```python
from build123d import *

# Parameters (mm, degrees)
BASE_SKETCH_W            = 254
BASE_SKETCH_H            = 304.8
BASE_DEPTH               = 25.4
RIGHT_TRIANGLE_DEPTH     = 25.4
LEFT_TRIANGLE_DEPTH      = 25.4
SUPPORT_BEAMS_SKETCH_W   = 114.3
SUPPORT_BEAMS_SKETCH_H   = 203.2
SUPPORT_BEAMS_SKETCH_W_2 = 50.8
SUPPORT_BEAMS_SKETCH_W_3 = 88.9
SUPPORT_BEAMS_DEPTH      = 25.4
FILLET1_R                = 12.7
TOP_PLATE_SKETCH_W       = 228.6
TOP_PLATE_SKETCH_H       = 254
TOP_PLATE_DEPTH          = 25.4
FILLET4_R                = 2.54
CUT_EXTRUDE1_DEPTH       = 229.6
FILLET6_R                = 6.35


with BuildPart() as part:
    # Base Sketch → Base (new body)
    with BuildSketch(Plane(origin=(0, 0, 0), x_dir=(0, 0, -1), z_dir=(1, 0, 0))):
        Rectangle(BASE_SKETCH_W, BASE_SKETCH_H)
    extrude(amount=BASE_DEPTH)

    # Right Triangle Sketch → Right Triangle (add)
    with BuildSketch(Plane.XY.offset(101.6)):
        Polygon((0, 152.4), (876.3, 152.4), (876.3, 127), (50.8, -152.4), (0, -152.4), align=None)
    extrude(amount=-RIGHT_TRIANGLE_DEPTH)

    # Left Triangle Sketch → Left Triangle (add)
    with BuildSketch(Plane(origin=(0, 0, -101.6), x_dir=(-1, 0, 0), z_dir=(0, 0, -1))):
        Polygon((0, 152.4), (-876.3, 152.4), (-876.3, 127), (-50.8, -152.4), (0, -152.4), align=None)
    extrude(amount=-LEFT_TRIANGLE_DEPTH)

    # Support Beams Sketch → Support Beams (add)
    with BuildSketch(Plane(origin=(0, 152.4, 0), x_dir=(1, 0, 0), z_dir=(0, 1, 0))):
        with Locations((57.15, 0)):
            Rectangle(SUPPORT_BEAMS_SKETCH_W, SUPPORT_BEAMS_SKETCH_H)
        with Locations((304.8, 0)):
            Rectangle(SUPPORT_BEAMS_SKETCH_W_2, SUPPORT_BEAMS_SKETCH_H)
        with Locations((831.85, 0)):
            Rectangle(SUPPORT_BEAMS_SKETCH_W_3, SUPPORT_BEAMS_SKETCH_H)
    extrude(amount=-SUPPORT_BEAMS_DEPTH)

    # Fillet1
    fillet1_edges = [part.edges().sort_by_distance(p)[0] for p in [
        (279.4, 139.7, 76.2),
        (330.2, 139.7, 76.2),
        (304.8, 127, 76.2),
        (304.8, 127, -76.2),
        (279.4, 139.7, -76.2),
        (330.2, 139.7, -76.2),
        (787.4, 139.7, 76.2),
        (831.85, 127, 76.2),
        (831.85, 127, -76.2),
        (787.4, 139.7, -76.2),
        (25.4, 0, 101.6),
        (876.3, 139.7, 101.6),
        (876.3, 139.7, -101.6),
        (25.4, 0, -101.6),
        (25.4, -12.7, -76.2),
        (25.4, -12.7, 76.2),
        (114.3, 139.7, 76.2),
        (69.85, 127, 76.2),
        (114.3, 139.7, -76.2),
        (25.4, 127, 0),
        (69.85, 127, -76.2),
    ]]
    fillet(fillet1_edges, radius=FILLET1_R)

    # Top Plate Sketch → Top Plate (add)
    with BuildSketch(Plane(origin=(0, 152.4, 0), x_dir=(1, 0, 0), z_dir=(0, 1, 0))):
        with Locations((698.5, 0)):
            Rectangle(TOP_PLATE_SKETCH_W, TOP_PLATE_SKETCH_H)
    extrude(amount=TOP_PLATE_DEPTH)

    # Fillet4
    fillet4_edges = [part.edges().sort_by_distance(p)[0] for p in [
        (787.4, 152.4, 0),
        (679.45, 152.4, 76.2),
        (783.680256121, 152.4, 72.480256121),
        (783.680256121, 152.4, -72.480256121),
        (679.45, 152.4, -76.2),
    ]]
    fillet(fillet4_edges, radius=FILLET4_R)

    # Sketch1 → Cut-Extrude1 (cut, through all)
    with BuildSketch(Plane.XY.offset(101.6)):
        Polygon((88.9, 12.7), (88.9, 114.3), (190.5, 114.3), align=None)
        Polygon((197.365304783, 49.323255814), (262.342048969, 114.3), (389.342048969, 114.3), align=None)
    extrude(amount=-CUT_EXTRUDE1_DEPTH, mode=Mode.SUBTRACT)

    # Fillet6
    fillet6_edges = [part.edges().sort_by_distance(p)[0] for p in [
        (190.5, 114.3, -88.9),
        (88.9, 12.7, -88.9),
        (88.9, 114.3, -88.9),
        (190.5, 114.3, 88.9),
        (88.9, 12.7, 88.9),
        (88.9, 114.3, 88.9),
        (389.342048969, 114.3, -88.9),
        (197.365304783, 49.323255814, -88.9),
        (262.342048969, 114.3, -88.9),
        (389.342048969, 114.3, 88.9),
        (197.365304783, 49.323255814, 88.9),
        (262.342048969, 114.3, 88.9),
    ]]
    fillet(fillet6_edges, radius=FILLET6_R)


solid = part.part
```
For this review, take the finished solid that the model builds, in its own axes (mm). A direction names the side the tool comes from. Give positions to 0.01 mm unless a question says otherwise; leave off trailing zeros. Loops run counter-clockwise (first coordinate to the right, second up) from the corner with the lowest first, then second, coordinate; pieces in that order, holes last. Notation, with made-up numbers: M 51,-25 L 75,-25 A19 ccw 75,7 Z; hole C 70,71 d6. An arc over 180 degrees is marked long. One line per item, written item: value. Start each with the question number.
Q1. Machinability: for faces 1 (the face through (844, 152.4, 1)), 2 (the face through (135, 114.3, 89)), 3 (the face through (831, 127, -1)), which of the approach directions +Z, -Z, +X, -X, +Y, -Y give a long, thin tool a straight path to every point of the face, cutting with its end or side? Answer none if there is none.
Q2. Clearance check with flat-ended pins moving along their axes: pin 1 Ø12 at (x, y) = (626, 51.5) entering from -Z; pin 2 Ø1 at (x, y) = (666, 84) entering from +Z; pin 3 Ø10 at (y, z) = (67.5, -119) entering from +X. State where each tip first meets the part, or that it passes through.
Q3. Add section C-C (z = 38). Give the boundary of the cut face in (x, y).
Q4. For L1, parallel to Z at x = 155, y = -65.5; L2, parallel to X at y = 145.5, z = 66.5; L3, parallel to Y at x = 788.5, z = -27, list the stretches that pass through material, from the lowest coordinate up.
Q5. Add section A-A (y = 141.5). Give the boundary of the cut face in (x, z).
Q6. Add section B-B (x = 482.5). Give the boundary of the cut face in (y, z).
Q7. Add section D-D (x = 751). Give the boundary of the cut face in (y, z), and give its area (3 significant figures).
Q8. Draft analysis for pull direction Y (two halves, no side actions). For faces 4 (the face through (876.3, 140, 1)), 5 (the face through (683, 152.4, -1)), 6 (the face through (140.3, 64.1, 89.1)), 7 (the face through (238.226, 90.184, 89.078)), state which applies: released by +Y, released by -Y, zero draft, split by the parting line, or undercut.
Reply:
1. face 1: +Z, -Z, +X, +Y
1. face 2: +Z, -Z
1. face 3: +X, -Y
2. pin 1: z = -101.6
2. pin 2: z = 101.6
2. pin 3: x = 25.4
3. outline: M 0,-152.4 L 25.4,-152.4 L 25.4,114.3 A12.7 cw 38.1,127 L 114.3,127 L 114.3,152.4 L 0,152.4 Z; M 279.4,127 L 330.2,127 L 330.2,152.4 L 279.4,152.4 Z; M 584.2,152.4 L 784.86,152.4 A2.54 cw 787.4,149.86 L 787.4,127 L 876.3,127 L 876.3,152.4 L 812.8,152.4 L 812.8,177.8 L 584.2,177.8 Z
4. L1: -101.6 to -76.2, 76.2 to 101.6
4. L2: 0 to 114.66, 279.04 to 330.56, 787.04 to 876.3
4. L3: 127 to 177.8
5. outline: M 0,-127 L 25.4,-127 L 25.4,-114.3 A12.7 cw 38.1,-101.6 L 863.6,-101.6 A12.7 ccw 876.3,-88.9 L 876.3,88.9 A12.7 ccw 863.6,101.6 L 38.1,101.6 A12.7 cw 25.4,114.3 L 25.4,127 L 0,127 Z; hole M 114.3,-63.5 A12.7 ccw 127,-76.2 L 266.7,-76.2 A12.7 ccw 279.4,-63.5 L 279.4,63.5 A12.7 ccw 266.7,76.2 L 127,76.2 A12.7 ccw 114.3,63.5 Z; hole M 330.2,-63.5 A12.7 ccw 342.9,-76.2 L 774.7,-76.2 A12.7 ccw 787.4,-63.5 L 787.4,63.5 A12.7 ccw 774.7,76.2 L 342.9,76.2 A12.7 ccw 330.2,63.5 Z
6. outline: M -6.29,-101.6 L 152.4,-101.6 L 152.4,-76.2 L -6.29,-76.2 Z; M -6.29,76.2 L 152.4,76.2 L 152.4,101.6 L -6.29,101.6 Z
7. outline: M 84.59,-101.6 L 152.4,-101.6 L 152.4,-127 L 177.8,-127 L 177.8,127 L 152.4,127 L 152.4,101.6 L 84.59,101.6 L 84.59,76.2 L 149.86,76.2 A2.54 cw 152.4,73.66 L 152.4,-73.66 A2.54 cw 149.86,-76.2 L 84.59,-76.2 Z
7. area: 9,900 mm²
8. face 4: zero draft
8. face 5: released by -Y
8. face 6: undercut
8. face 7: undercut
